Check sheet for the modelled part. Datum: model origin and axes. Units: mm. A direction names the side the tool comes from. Give positions to 0.01 mm unless a question says otherwise; leave off trailing zeros. Loops run counter-clockwise (first coordinate to the right, second up) from the corner with the lowest first, then second, coordinate; pieces in that order, holes last. Notation, with made-up numbers: M 69,-9.5 L 83,-9.5 A28 cw 83,20.5 Z; hole C -3.75,61.25 d3. An arc over 180 degrees is marked long. One line per question, with ' | ' between items. Start each with the question number.
from build123d import *

# Parameters (mm, degrees)
CYLINDER045_W               = 5.5
CYLINDER045_H               = 4.8
CYLINDER045_ANGLE           = 84
CYLINDER045_PLACEMENT_ANGLE = 3
FILLET004_R                 = 0.79
ARRAY008_COUNT              = 4
CYLINDER049_R               = 3.9
CYLINDER049_DEPTH           = 10
CYLINDER048_R               = 1.5
CYLINDER048_DEPTH           = 10
ARRAY010_X_COUNT            = 2
ARRAY010_X_PITCH            = 21
ARRAY010_Y_COUNT            = 2
ARRAY010_Y_PITCH            = 8
BOX007_W                    = 3
BOX007_H                    = 12.9
BOX007_DEPTH                = 10
BOX006_W                    = 3
BOX006_H                    = 13.9
BOX006_DEPTH                = 10
CYLINDER061_R               = 0.5
CYLINDER061_DEPTH           = 10
ARRAY015_COUNT              = 4
ARRAY015_PLACEMENT_ANGLE    = 28
BOX004_W                    = 25
BOX004_H                    = 12
BOX004_DEPTH                = 4
FILLET006_R                 = 2
BOX009_W                    = 30
BOX009_H                    = 18
BOX009_DEPTH                = 10


with BuildPart() as array008:
    # Cylinder045 → Cylinder045 (revolve)
    with BuildSketch(Plane.XZ):
        with Locations((2.75, 2.4)):
            Rectangle(CYLINDER045_W, CYLINDER045_H)
    revolve(axis=Axis((0, 0, 0), (0, 0, 1)), revolution_arc=CYLINDER045_ANGLE)


with BuildPart() as array008_1:
    # Cylinder045 placement: moved
    add(array008.part.moved(Location((0, 0, 0.6))).rotate(Axis((0, 0, 0.6), (0, 0, 1)), CYLINDER045_PLACEMENT_ANGLE))

    # Fillet004
    fillet004_edges = [array008_1.edges().sort_by_distance(p)[0] for p in [
        (0.287848, 5.492462, 3),
        (5.492462, 0.287848, 3),
    ]]
    fillet(fillet004_edges, radius=FILLET004_R)

    # Array008: Array008 ×4 about axis
    array008_axis = Axis((0, 0, 0), (0, 0, 1))


with BuildPart() as array008_2:
    add(array008_1.part)
    for i in range(1, ARRAY008_COUNT):
        add(array008_1.part.rotate(array008_axis, i * 360 / ARRAY008_COUNT))


with BuildPart() as mountplateinnerhole003:
    # Cylinder049 → Cylinder049 (new body)
    with BuildSketch(Plane.XY):
        Circle(CYLINDER049_R)
    extrude(amount=CYLINDER049_DEPTH)


with BuildPart() as array010:
    # Cylinder048 → Cylinder048 (new body)
    with BuildSketch(Plane.XY):
        Circle(CYLINDER048_R)
    extrude(amount=CYLINDER048_DEPTH)

    # Array010 X: Array010 ×2


with BuildPart() as array010_1:
    add(array010.part)
    with Locations(*[(i * ARRAY010_X_PITCH, 0, 0) for i in range(1, ARRAY010_X_COUNT)]):
        add(array010.part)

    # Array010 Y: Array010 ×2


with BuildPart() as array010_2:
    add(array010_1.part)
    with Locations(*[(0, i * ARRAY010_Y_PITCH, 0) for i in range(1, ARRAY010_Y_COUNT)]):
        add(array010_1.part)


with BuildPart() as array010_3:
    # Array010 placement: moved
    add(array010_2.part.moved(Location((-10.5, -4, 0))))


with BuildPart() as cube007:
    # Box007 → Box007 (new body)
    with BuildSketch(Plane(origin=(-9.1, -6, 2), x_dir=(1, 0, 0), z_dir=(0, 0, 1))):
        with Locations((1.5, 6.45)):
            Rectangle(BOX007_W, BOX007_H)
    extrude(amount=BOX007_DEPTH)


with BuildPart() as cube006:
    # Box006 → Box006 (new body)
    with BuildSketch(Plane(origin=(6.1, -7, 2), x_dir=(1, 0, 0), z_dir=(0, 0, 1))):
        with Locations((1.5, 6.95)):
            Rectangle(BOX006_W, BOX006_H)
    extrude(amount=BOX006_DEPTH)


with BuildPart() as fusion019:
    # Cylinder061 → Cylinder061 (new body)
    with BuildSketch(Plane(origin=(6, 2, 0), x_dir=(1, 0, 0), z_dir=(0, 0, 1))):
        Circle(CYLINDER061_R)
    extrude(amount=CYLINDER061_DEPTH)

    # Array015: Fusion019 ×4 about axis
    array015_axis = Axis((0, 0, 0), (0, 0, 1))


with BuildPart() as fusion019_1:
    add(fusion019.part)
    for i in range(1, ARRAY015_COUNT):
        add(fusion019.part.rotate(array015_axis, i * 360 / ARRAY015_COUNT))


with BuildPart() as fusion019_2:
    # Array015 placement: moved
    add(fusion019_1.part.rotate(Axis((0, 0, 0), (0, 0, 1)), ARRAY015_PLACEMENT_ANGLE))

    # Fusion019: union Array008, MountPlateInnerHole003, Array010, Cube007, Cube006
    add(array008_2.part)
    add(mountplateinnerhole003.part)
    add(array010_3.part)
    add(cube007.part)
    add(cube006.part)


with BuildPart() as frontplate:
    # Box004 → Box004 (new body)
    with BuildSketch(Plane(origin=(-12.5, -6, 0), x_dir=(1, 0, 0), z_dir=(0, 0, 1))):
        with Locations((12.5, 6)):
            Rectangle(BOX004_W, BOX004_H)
    extrude(amount=BOX004_DEPTH)

    # Fillet006
    fillet006_edges = [frontplate.edges().sort_by_distance(p)[0] for p in [
        (-12.5, -6, 2),
        (-12.5, 6, 2),
        (12.5, -6, 2),
        (12.5, 6, 2),
    ]]
    fillet(fillet006_edges, radius=FILLET006_R)

    # Cut022: cut Fusion019
    add(fusion019_2.part, mode=Mode.SUBTRACT)


with BuildPart() as cut024:
    # Box009 → Box009 (new body)
    with BuildSketch(Plane(origin=(-15, -9, 0), x_dir=(1, 0, 0), z_dir=(0, 0, 1))):
        with Locations((15, 9)):
            Rectangle(BOX009_W, BOX009_H)
    extrude(amount=BOX009_DEPTH)

    # Cut024: cut FrontPlate
    add(frontplate.part, mode=Mode.SUBTRACT)


solid = cut024.part
Q1. Material ranges on probe 1 along Y at (x, z) = (11.25, 3); probe 2 along X at (y, z) = (2, 2.5); probe 3 along Y at (x, z) = (3.25, 1.75), recorded low to high. Write a range as from..to.
Q2. Depth check by flat-ended pin: P1, Ø2.5, axis at x = 10.5, y = 1, coming from the -Z side; P2, Ø0.9, axis at x = 7.5, y = 0, coming from the -Z side. Enter the tip coordinate at first touch or a pass-through.
Q3. Cross-section at A-A (y = 2). Record the cut outline in (x, z), and give its area (3 significant figures).
Q4. Draft check along Y on faces 1 (the cylindrical face through (-12, -4, 2)), 2 (the flat face through (0, -9, 5)), 3 (the flat face through (-11, -4, 0)). Enter one of: released by +Y, released by -Y, zero draft, split by the parting line, or undercut.
Q5. Cross-section at B-B (x = 1.5). Record the cut outline in (y, z), and give its area (3 significant figures).
Q6. Access from +Z, -Z, +X, -X, +Y, -Y to the whole of each face (thin tool, end or side, straight path). Record for faces 4 (the flat face through (-15, 0, 5)), 5 (the cylindrical face through (5.23, 0.56, 2.32)).
Solved:
1) probe 1: y = -9..-5.85, -5.3..-2.7, 2.7..5.3, 5.85..9 | probe 2: x = -15..-12.5, -9.1..-6.1, -5.12..5.12, 6.1..9.1, 12.5..15 | probe 3: y = -9..-6, -4.44..4.44, 6..9
2) P1: stops at z = 4 | P2: stops at z = 2
3) outline: M -15,0 L -12.5,0 L -12.5,4 L -9.1,4 L -9.1,2 L -6.1,2 L -6.1,4 L -5.12,4 L -5.12,0.6 L -3.35,0.6 L -3.35,0 L 3.35,0 L 3.35,0.6 L 5.12,0.6 L 5.12,4 L 6.1,4 L 6.1,2 L 9.1,2 L 9.1,4 L 12.5,4 L 12.5,0 L 15,0 L 15,10 L -15,10 Z | area: 251 mm²
4) face 1: undercut | face 2: released by -Y | face 3: zero draft
5) outline: M -9,0 L -6,0 L -6,4 L -5.29,4 L -5.29,0.6 L -3.6,0.6 L -3.6,0 L 3.6,0 L 3.6,0.6 L 5.29,0.6 L 5.29,4 L 6,4 L 6,0 L 9,0 L 9,10 L -9,10 Z | area: 172 mm²
6) face 4: +Z, -Z, -X, +Y, -Y | face 5: -Z
